Could you check a few things on this model? Use its own coordinates, in mm. A direction names the side the tool comes from. Give positions to 0.01 mm unless a question says otherwise; leave off trailing zeros. Loops run counter-clockwise (first coordinate to the right, second up) from the corner with the lowest first, then second, coordinate; pieces in that order, holes last. Notation, with made-up numbers: (52, -9) -> (98, -9) arc R21 ccw to (98, 29) -> close; hole circle Ø2 at (12.5, -10.5). An arc over 180 degrees is marked (long way). Write each question's results on one line, items separated by ' | '. Start each with the question number.
Q1. If we section it at B-B, the plane y = 5.25: List the corners of the cut face in (x, z) for me (1 decimal).
Q2. Which directions (+Z, -Z, +X, -X, +Y, -Y) give clear straight access to the entire face, cutting with the end or side of a thin tool? Please do faces 1 (the face through (2.41, 3.13, 9.95)), 2 (the face through (16.11, 3.12, 2.35)).
Q3. If we section it at A-A, the plane x = 9.25: List the corners of the cut face in (y, z) for me.
Q4. Will these pins go through, and if not, where does the flat tip stop? P1, Ø2.5, axis at x = 17.46, y = 3.18, coming from the -Z side; P2, Ø2.5, axis at x = 3.175, y = 3.175, coming from the +Z side (3 decimals).
Q5. If we section it at D-D, the plane x = 18: List the corners of the cut face in (y, z) for me.
Q6. We'd pull the mould along Y, two halves only. Please class faces 3 (the face through (17, 3, 4.762)), 4 (the face through (3, 3, 4.762)), 5 (the face through (10, 3, 0)), 6 (the face through (10, 6.35, 6)): released by +Y, released by -Y, zero draft, split by the parting line, or undercut.
Q7. If I drill on line 1 along X through (y, z) = (1.75, 9); line 2 along Y through (x, z) = (3.25, 1); line 3 along X through (y, z) = (4, 4.5), over which ranges is the centre line in solid material (lowest first)?
Q8. If we section it at C-C, the plane z = 7.75: List the corners of the cut face in (x, y) for me, plus the area to 3 significant figures.
from build123d import *

# Parameters (mm, degrees)
F0_W     = 20.6375
F0_H     = 6.35
F1_DEPTH = 12.30249
F2_R     = 1.7272
F3_DEPTH = 6.35
F4_R     = 1.35255
F5_DEPTH = 4.7625
F6_SIZE  = 4.7625


with BuildPart() as f1:
    # F0 (on Top) → F1 (new body)
    with BuildSketch(Plane.XY):
        with Locations((10.31875, 3.175)):
            Rectangle(F0_W, F0_H)
    extrude(amount=F1_DEPTH)

    # F2 (on face) → F3 (cut, through all)
    with BuildSketch(Plane.XZ):
        with Locations((10.31875, 8.33374)):
            Circle(F2_R)
    extrude(amount=-F3_DEPTH, mode=Mode.SUBTRACT)

    # F4 (on face) → F5 (cut)
    with BuildSketch(Plane(origin=(0, 0, 0), x_dir=(1, 0, 0), z_dir=(0, 0, -1))):
        with Locations((3.175, -3.175)):
            Circle(F4_R)
        with Locations((17.4625, -3.175)):
            Circle(F4_R)
    extrude(amount=-F5_DEPTH, mode=Mode.SUBTRACT)

    # F6
    f6_edges = [f1.edges().sort_by_distance(p)[0] for p in [
        (0, 3.175, 12.30249),
        (20.6375, 3.175, 12.30249),
    ]]
    chamfer(f6_edges, length=F6_SIZE)


solid = f1.part
Final values:
1) outline: (0, 0) -> (20.6, 0) -> (20.6, 7.5) -> (15.9, 12.3) -> (4.8, 12.3) -> (0, 7.5) -> close; hole circle Ø3.5 at (10.3, 8.3)
2) face 1: +Z, -X, +Y, -Y | face 2: -Z
3) outline: (0, 0) -> (6.35, 0) -> (6.35, 6.98) -> (0, 6.98) -> close; (0, 9.69) -> (6.35, 9.69) -> (6.35, 12.3) -> (0, 12.3) -> close
4) P1: stops at z = 4.76 | P2: stops at z = 11.965
5) outline: (0, 0) -> (1.93, 0) -> (1.93, 4.76) -> (4.42, 4.76) -> (4.42, 0) -> (6.35, 0) -> (6.35, 10.18) -> (0, 10.18) -> close
6) face 3: undercut | face 4: undercut | face 5: zero draft | face 6: released by +Y
7) line 1: x = 1.46 to 8.73, 11.91 to 19.18 | line 2: y = 0 to 1.82, 4.53 to 6.35 | line 3: x = 0 to 2.1, 4.25 to 16.39, 18.53 to 20.64
8) outline: (0.21, 0) -> (8.69, 0) -> (8.69, 6.35) -> (0.21, 6.35) -> close; (11.94, 0) -> (20.43, 0) -> (20.43, 6.35) -> (11.94, 6.35) -> close | area: 108 mm²
